```python
from build123d import *

# Parameters (mm, degrees)
F2_R      = 139.7
F3_DEPTH  = 19.05
F4_SIZE   = 1.5875
F5_R      = 0.79375
F6_DEPTH  = 19.051
F7_R      = 2.9765625
F7_R_2    = 0.79375
F8_DEPTH  = 19.051
F9_R      = 2.9765625
F10_DEPTH = 19.051
F11_R     = 9.525
F11_R_2   = 2.9765625
F12_DEPTH = 6.35
F13_R     = 3.175
F14_DEPTH = 19.051
F15_R     = 1.1938
F16_DEPTH = 12.7
F17_R     = 7.9375
F17_R_2   = 3.175
F17_R_3   = 1.1938
F18_DEPTH = 10.16
F19_R     = 4.7625
F19_R_2   = 3.175
F20_DEPTH = 4.7752


# Not quite as in the source:
# - a variable given as a bare number and used for a length is read in inches; the dataset says mm whatever the document's units were


with BuildPart() as f3:
    # F2 (on Top) → F3 (new body)
    with BuildSketch(Plane.XY):
        Circle(F2_R)
    extrude(amount=F3_DEPTH)

    # F4
    f4_edges = [f3.edges().sort_by_distance(p)[0] for p in [
        (-139.7, 0, 19.05),
        (-139.7, 0, 0),
    ]]
    chamfer(f4_edges, length=F4_SIZE)

    # F5 (on face) → F6 (cut, through all)
    with BuildSketch(Plane.XY.offset(19.05)):
        with Locations((-92.047625241, 92.047625241)):
            Circle(F5_R)
        with Locations((92.047625241, 92.047625241)):
            Circle(F5_R)
        with Locations((92.047625241, -92.047625241)):
            Circle(F5_R)
        with Locations((-92.047625241, -92.047625241)):
            Circle(F5_R)
    extrude(amount=-F6_DEPTH, mode=Mode.SUBTRACT)

    # F7 (on face) → F8 (cut, through all)
    with BuildSketch(Plane.XY.offset(19.05)):
        with Locations((-92.047625241, 92.047625241)):
            Circle(F7_R)
        with Locations((-92.047625241, 92.047625241)):
            Circle(F7_R_2, mode=Mode.SUBTRACT)
        with Locations((92.047625241, 92.047625241)):
            Circle(F7_R)
        with Locations((92.047625241, 92.047625241)):
            Circle(F7_R_2, mode=Mode.SUBTRACT)
        with Locations((-92.047625241, -92.047625241)):
            Circle(F7_R)
        with Locations((-92.047625241, -92.047625241)):
            Circle(F7_R_2, mode=Mode.SUBTRACT)
        with Locations((92.047625241, -92.047625241)):
            Circle(F7_R)
        with Locations((92.047625241, -92.047625241)):
            Circle(F7_R_2, mode=Mode.SUBTRACT)
    extrude(amount=-F8_DEPTH, mode=Mode.SUBTRACT)

    # F9 (on face) → F10 (cut, through all)
    with BuildSketch(Plane.XY.offset(19.05)):
        with Locations((0, 107.95)):
            Circle(F9_R)
        with Locations((107.95, 0)):
            Circle(F9_R)
        with Locations((0, -107.95)):
            Circle(F9_R)
        with Locations((-107.95, 0)):
            Circle(F9_R)
    extrude(amount=-F10_DEPTH, mode=Mode.SUBTRACT)

    # F11 (on face) → F12 (cut)
    with BuildSketch(Plane.XY.offset(19.05)):
        with Locations((0, 107.95)):
            Circle(F11_R)
        with Locations((0, 107.95)):
            Circle(F11_R_2, mode=Mode.SUBTRACT)
        with Locations((107.95, 0)):
            Circle(F11_R)
        with Locations((107.95, 0)):
            Circle(F11_R_2, mode=Mode.SUBTRACT)
        with Locations((0, -107.95)):
            Circle(F11_R)
        with Locations((0, -107.95)):
            Circle(F11_R_2, mode=Mode.SUBTRACT)
        with Locations((-107.95, 0)):
            Circle(F11_R)
        with Locations((-107.95, 0)):
            Circle(F11_R_2, mode=Mode.SUBTRACT)
    extrude(amount=-F12_DEPTH, mode=Mode.SUBTRACT)

    # F13 (on face) → F14 (cut, through all)
    with BuildSketch(Plane.XY.offset(19.05)):
        with Locations((36.921074472, 101.4398184138)):
            Circle(F13_R)
        with Locations((53.975, 93.4874423385)):
            Circle(F13_R)
        with Locations((69.3889224657, 82.6944976347)):
            Circle(F13_R)
        with Locations((82.6944976347, 69.3889224657)):
            Circle(F13_R)
        with Locations((93.4874423385, 53.975)):
            Circle(F13_R)
        with Locations((101.4398184138, 36.921074472)):
            Circle(F13_R)
    extrude(amount=-F14_DEPTH, mode=Mode.SUBTRACT)

    # F15 (on face) → F16 (cut)
    with BuildSketch(Plane(origin=(0, 0, 0), x_dir=(1, 0, 0), z_dir=(0, 0, -1))):
        with Locations((50.927, -88.2081514771)):
            Circle(F15_R)
        with Locations((65.470489197, -78.0246907094)):
            Circle(F15_R)
        with Locations((78.0246907094, -65.470489197)):
            Circle(F15_R)
        with Locations((88.2081514771, -50.927)):
            Circle(F15_R)
        with Locations((95.7114521975, -34.8361196783)):
            Circle(F15_R)
        with Locations((34.8361196783, -95.7114521975)):
            Circle(F15_R)
    extrude(amount=-F16_DEPTH, mode=Mode.SUBTRACT)

    # F17 (on face) → F18 (cut)
    with BuildSketch(Plane(origin=(0, 0, 0), x_dir=(1, 0, 0), z_dir=(0, 0, -1))):
        with Locations((36.921074472, -101.4398184138)):
            Circle(F17_R)
        with Locations((36.921074472, -101.4398184138)):
            Circle(F17_R_2, mode=Mode.SUBTRACT)
        with Locations((34.8361196783, -95.7114521975)):
            Circle(F17_R_3, mode=Mode.SUBTRACT)
        with Locations((53.975, -93.4874423385)):
            Circle(F17_R)
        with Locations((50.927, -88.2081514771)):
            Circle(F17_R_3, mode=Mode.SUBTRACT)
        with Locations((53.975, -93.4874423385)):
            Circle(F17_R_2, mode=Mode.SUBTRACT)
        with Locations((69.3889224657, -82.6944976347)):
            Circle(F17_R)
        with Locations((65.470489197, -78.0246907094)):
            Circle(F17_R_3, mode=Mode.SUBTRACT)
        with Locations((69.3889224657, -82.6944976347)):
            Circle(F17_R_2, mode=Mode.SUBTRACT)
        with Locations((82.6944976347, -69.3889224657)):
            Circle(F17_R)
        with Locations((82.6944976347, -69.3889224657)):
            Circle(F17_R_2, mode=Mode.SUBTRACT)
        with Locations((78.0246907094, -65.470489197)):
            Circle(F17_R_3, mode=Mode.SUBTRACT)
        with Locations((93.4874423385, -53.975)):
            Circle(F17_R)
        with Locations((93.4874423385, -53.975)):
            Circle(F17_R_2, mode=Mode.SUBTRACT)
        with Locations((88.2081514771, -50.927)):
            Circle(F17_R_3, mode=Mode.SUBTRACT)
        with Locations((101.4398184138, -36.921074472)):
            Circle(F17_R)
        with Locations((95.7114521975, -34.8361196783)):
            Circle(F17_R_3, mode=Mode.SUBTRACT)
        with Locations((101.4398184138, -36.921074472)):
            Circle(F17_R_2, mode=Mode.SUBTRACT)
    extrude(amount=-F18_DEPTH, mode=Mode.SUBTRACT)

    # F19 (on face) → F20 (cut)
    with BuildSketch(Plane.XY.offset(19.05)):
        with Locations((36.921074472, 101.4398184138)):
            Circle(F19_R)
        with Locations((36.921074472, 101.4398184138)):
            Circle(F19_R_2, mode=Mode.SUBTRACT)
        with Locations((53.975, 93.4874423385)):
            Circle(F19_R)
        with Locations((53.975, 93.4874423385)):
            Circle(F19_R_2, mode=Mode.SUBTRACT)
        with Locations((69.3889224657, 82.6944976347)):
            Circle(F19_R)
        with Locations((69.3889224657, 82.6944976347)):
            Circle(F19_R_2, mode=Mode.SUBTRACT)
        with Locations((82.6944976347, 69.3889224657)):
            Circle(F19_R)
        with Locations((82.6944976347, 69.3889224657)):
            Circle(F19_R_2, mode=Mode.SUBTRACT)
        with Locations((93.4874423385, 53.975)):
            Circle(F19_R)
        with Locations((93.4874423385, 53.975)):
            Circle(F19_R_2, mode=Mode.SUBTRACT)
        with Locations((101.4398184138, 36.921074472)):
            Circle(F19_R)
        with Locations((101.4398184138, 36.921074472)):
            Circle(F19_R_2, mode=Mode.SUBTRACT)
    extrude(amount=-F20_DEPTH, mode=Mode.SUBTRACT)


solid = f3.part
```
Could you check a few things on this model? Use its own coordinates, in mm. A direction names the side the tool comes from. Coordinates: 2 decimals unless noted, no trailing zeros. One line per question, with ' | ' between items. Start each with the question number.
1. For faces 4 (the face through (34.581, 103.586, 12.246)), 5 (the face through (97, 54, 10.16)), 6 (the face through (73.93, 84.13, 16.7)), which set-ups out of +Z, -Z, +X, -X, +Y, -Y let a thin tool reach every point of the face, with its end or its side?
2. Thinking about a two-plate mould opening in Y: for faces 1 (the face through (-110.2, 2.3, 12.7)), 2 (the face through (-2, 2, 0)), 3 (the face through (-110.86, -85.01, 9.41)), which applies, pulls with the +Y half, pulls with the -Y half, needs draft (parallel to the pull), parting line crosses it, or undercut?
3. Will these pins go through, and if not, where does the flat tip stop? P1, Ø2.5, axis at x = 88.5, y = 50.5, coming from the -Z side; P2, Ø3, axis at x = 81, y = 67.5, coming from the +Z side; P3, Ø5.5, axis at x = 107.5, y = 0, coming from the +Z side.
4. Please list where these lines run through material, in increasing order: line 1 along Y through (x, z) = (0, 14.75) (3 decimals); line 2 along X through (y, z) = (95.5, 2.25); line 3 along X through (y, z) = (3.5, 17.25).
5. If we section it at A-A (z = 5.5): Count the separate pieces of the cut face and the enclosed holes in it, and give its area (3 significant figures).
Return value:
1) face 4: +Z, -Z | face 5: -Z | face 6: +Z
2) face 1: undercut | face 2: needs draft | face 3: parting line crosses it
3) P1: stops at z = 10.16 | P2: stops at z = 14.27 | P3: stops at z = 12.7
4) line 1: y = -139.7 to -117.475, -98.425 to 98.425, 117.475 to 139.7 | line 2: x = -101.96 to 31.66, 42.19 to 46.3, 61.65 to 101.96 | line 3: x = -139.66 to -116.81, -99.09 to 99.09, 116.81 to 139.66
5) separate pieces: 1 | enclosed holes: 14 | area: 59,900 mm²
